from build123d import *

# Parameters (mm, degrees)
SKETCH1_W                    = 62.75
SKETCH1_H                    = 45.15
BOSS_EXTRUDE1_DEPTH          = 23.4
SKETCH2_W                    = 30
SKETCH2_H                    = 42.9
CUT_EXTRUDE1_DEPTH           = 0.95
SKETCH3_W                    = 15
SKETCH3_H                    = 13.4
CUT_EXTRUDE2_DEPTH           = 4.3
SKETCH4_R                    = 3.5
BOSS_EXTRUDE2_DEPTH          = 3
CUT_EXTRUDE3_DEPTH           = 18.6
SKETCH6_W                    = 0.2
SKETCH6_H                    = 5
CUT_EXTRUDE_THIN1_DEPTH      = 1.95
CUT_EXTRUDE_THIN1_DEPTH_BACK = 1
CUT_EXTRUDE4_DEPTH           = 5.8
SKETCH8_R                    = 2.25
CUT_EXTRUDE5_DEPTH           = 5.8
SKETCH9_W                    = 1.525
SKETCH9_H                    = 45.15
CUT_EXTRUDE6_DEPTH           = 20
SKETCH11_W                   = 1.525
SKETCH11_H                   = 10.4
BOSS_EXTRUDE3_DEPTH          = 1.4
CHAMFER1_SIZE                = 1
SKETCH10_W                   = 3
SKETCH10_H                   = 8.15
CUT_EXTRUDE7_DEPTH           = 3.75


with BuildPart() as part:
    # Sketch1 → Boss-Extrude1 (new body)
    with BuildSketch(Plane(origin=(0, 0, 0), x_dir=(1, 0, 0), z_dir=(0, 1, 0))):
        Rectangle(SKETCH1_W, SKETCH1_H)
    extrude(amount=BOSS_EXTRUDE1_DEPTH)

    # Sketch2 → Cut-Extrude1 (cut)
    with BuildSketch(Plane(origin=(0, 23.4, 0), x_dir=(1, 0, 0), z_dir=(0, 1, 0))):
        Rectangle(SKETCH2_W, SKETCH2_H)
    extrude(amount=-CUT_EXTRUDE1_DEPTH, mode=Mode.SUBTRACT)

    # Sketch3 → Cut-Extrude2 (cut)
    with BuildSketch(Plane(origin=(0, 23.4, 0), x_dir=(1, 0, 0), z_dir=(0, 1, 0))):
        with Locations((-23.875, 12.925)):
            Rectangle(SKETCH3_W, SKETCH3_H)
        with Locations((-23.875, -12.925)):
            Rectangle(SKETCH3_W, SKETCH3_H)
        with Locations((23.875, -12.925)):
            Rectangle(SKETCH3_W, SKETCH3_H)
        with Locations((23.875, 12.925)):
            Rectangle(SKETCH3_W, SKETCH3_H)
    extrude(amount=-CUT_EXTRUDE2_DEPTH, mode=Mode.SUBTRACT)

    # Sketch4 → Boss-Extrude2 (add)
    with BuildSketch(Plane(origin=(0, 19.1, 0), x_dir=(1, 0, 0), z_dir=(0, 1, 0))):
        with Locations((-23.875, 12.925)):
            Circle(SKETCH4_R)
        with Locations((-23.875, -12.925)):
            Circle(SKETCH4_R)
        with Locations((23.875, -12.925)):
            Circle(SKETCH4_R)
        with Locations((23.875, 12.925)):
            Circle(SKETCH4_R)
    extrude(amount=BOSS_EXTRUDE2_DEPTH)

    # Sketch5 → Cut-Extrude3 (cut)
    with BuildSketch(Plane(origin=(0, 23.4, 0), x_dir=(1, 0, 0), z_dir=(0, 1, 0))):
        with BuildLine():
            Line((31.375, -5.2), (23.175, -5.2))
            ThreePointArc((23.175, -5.2), (17.975, 0), (23.175, 5.2))
            Line((23.175, 5.2), (31.375, 5.2))
            ThreePointArc((31.375, 5.2), (36.575, 0), (31.375, -5.2))
        make_face()
        with BuildLine():
            Line((-31.375, 5.2), (-24.325, 5.2))
            ThreePointArc((-24.325, 5.2), (-19.125, 0), (-24.325, -5.2))
            Line((-24.325, -5.2), (-31.375, -5.2))
            ThreePointArc((-31.375, -5.2), (-36.575, 0), (-31.375, 5.2))
        make_face()
    extrude(amount=-CUT_EXTRUDE3_DEPTH, mode=Mode.SUBTRACT)

    # Sketch6 → Cut-Extrude-Thin1 (cut, two sides)
    with BuildSketch(Plane(origin=(0, 22.45, 0), x_dir=(1, 0, 0), z_dir=(0, 1, 0))) as cut_extrude_thin1_sk:
        with Locations((13.9, 0)):
            Rectangle(SKETCH6_W, SKETCH6_H)
    extrude(amount=CUT_EXTRUDE_THIN1_DEPTH, mode=Mode.SUBTRACT)
    extrude(cut_extrude_thin1_sk.sketch, amount=-CUT_EXTRUDE_THIN1_DEPTH_BACK, mode=Mode.SUBTRACT)

    # Sketch7 → Cut-Extrude4 (cut, through all)
    with BuildSketch(Plane(origin=(0, 4.8, 0), x_dir=(1, 0, 0), z_dir=(0, 1, 0))):
        with BuildLine():
            Line((22.275, 2.25), (25.075, 2.25))
            ThreePointArc((25.075, 2.25), (27.325, 0), (25.075, -2.25))
            Line((25.075, -2.25), (22.275, -2.25))
            ThreePointArc((22.275, -2.25), (20.025, 0), (22.275, 2.25))
        make_face()
    extrude(amount=-CUT_EXTRUDE4_DEPTH, mode=Mode.SUBTRACT)

    # Sketch8 → Cut-Extrude5 (cut, through all)
    with BuildSketch(Plane(origin=(0, 4.8, 0), x_dir=(1, 0, 0), z_dir=(0, 1, 0))):
        with Locations((-23.825, 0)):
            Circle(SKETCH8_R)
    extrude(amount=-CUT_EXTRUDE5_DEPTH, mode=Mode.SUBTRACT)

    # Sketch9 → Cut-Extrude6 (cut)
    with BuildSketch(Plane(origin=(0, 23.4, 0), x_dir=(1, 0, 0), z_dir=(0, 1, 0))):
        with Locations((-30.6125, 0)):
            Rectangle(SKETCH9_W, SKETCH9_H)
        with Locations((30.6125, 0)):
            Rectangle(SKETCH9_W, SKETCH9_H)
    extrude(amount=-CUT_EXTRUDE6_DEPTH, mode=Mode.SUBTRACT)

    # Sketch11 → Boss-Extrude3 (add)
    with BuildSketch(Plane(origin=(0, 3.4, 0), x_dir=(1, 0, 0), z_dir=(0, 1, 0))):
        with Locations((-30.6125, 0)):
            Rectangle(SKETCH11_W, SKETCH11_H)
        with Locations((30.6125, 0)):
            Rectangle(SKETCH11_W, SKETCH11_H)
    extrude(amount=BOSS_EXTRUDE3_DEPTH)

    # Chamfer1
    chamfer1_edges = [part.edges().sort_by_distance(p)[0] for p in [
        (-31.375, 4.8, 0),
        (31.375, 4.8, 0),
    ]]
    chamfer(chamfer1_edges, length=CHAMFER1_SIZE)

    # Sketch10 → Cut-Extrude7 (cut)
    with BuildSketch(Plane.XZ):
        with Locations((29.875, 0)):
            Rectangle(SKETCH10_W, SKETCH10_H)
        with Locations((-29.875, 0)):
            Rectangle(SKETCH10_W, SKETCH10_H)
    extrude(amount=-CUT_EXTRUDE7_DEPTH, mode=Mode.SUBTRACT)


solid = part.part
For this review, take the finished solid that the model builds, in its own axes (mm). A direction names the side the tool comes from. Coordinates: 2 decimals unless noted, no trailing zeros. Order: outer loops, then holes, each group sorted by start corner. A loop starts at its lowest first (then second) coordinate and runs counter-clockwise, first axis right, second up. Notation, with made-up numbers: (38, 1) -> (58, 1) arc R13 ccw to (58, 17) -> close; hole circle Ø4 at (75, 33.5). An arc over 180 degrees is marked (long way). Return JSON: item names as keys, results as strings.
1. We need section A-A on z = 0. State how many separate pieces and enclosed holes the cut face has, and give its area (3 significant figures).
Answer block:
{"separate pieces": "3", "enclosed holes": "0", "area": "882 mm²"}
2. We need section D-D on z = -10.5. Write out the cut boundary in (x, y) (3 decimals).
Answer block:
{"outline": "(-31.375, 0) -> (31.375, 0) -> (31.375, 3.4) -> (29.85, 3.4) -> (29.85, 19.1) -> (26.399, 19.1) -> (26.399, 22.1) -> (21.351, 22.1) -> (21.351, 19.1) -> (16.375, 19.1) -> (16.375, 23.4) -> (15, 23.4) -> (15, 22.45) -> (-15, 22.45) -> (-15, 23.4) -> (-16.375, 23.4) -> (-16.375, 19.1) -> (-21.351, 19.1) -> (-21.351, 22.1) -> (-26.399, 22.1) -> (-26.399, 19.1) -> (-29.85, 19.1) -> (-29.85, 3.4) -> (-31.375, 3.4) -> close"}
3. We need section B-B on y = 7.25. Write out the cut boundary in (x, z) (3 decimals), and give its area (3 significant figures).
Answer block:
{"outline": "(-29.85, -22.575) -> (29.85, -22.575) -> (29.85, -5.2) -> (23.175, -5.2) arc R5.2 cw to (23.175, 5.2) -> (29.85, 5.2) -> (29.85, 22.575) -> (-29.85, 22.575) -> (-29.85, 5.2) -> (-24.325, 5.2) arc R5.2 cw to (-24.325, -5.2) -> (-29.85, -5.2) -> close", "area": "2,480 mm²"}
4. The part is to be moulded in two halves that separate along Z. For faces 1 (the flat face through (0, 12, -22.575)), 2 (the cylindrical face through (17.976, 14.23, 0.114)), 3 (the flat face through (31, 3.4, 14)), say which applies: +Z half, -Z half, draft (parallel to the pull), parting line (faces both ways), or undercut.
Answer block:
{"face 1": "-Z half", "face 2": "undercut", "face 3": "draft"}
5. We need section C-C on x = 9.5. Write out the cut boundary in (y, z) (3 decimals).
Answer block:
{"outline": "(0, -22.575) -> (23.4, -22.575) -> (23.4, -21.45) -> (22.45, -21.45) -> (22.45, 21.45) -> (23.4, 21.45) -> (23.4, 22.575) -> (0, 22.575) -> close"}
6. For line 1 (X direction, y = 2.35, z = 0) (3 decimals); line 2 (Z direction, x = -25, y = 6) (3 decimals); line 3 (Z direction, x = 22, y = 21) (1 decimal), list the stretches that pass through material, from the lowest coordinate up. Write a range as from..to.
Answer block:
{"line 1": "-28.375..-26.075, -21.575..20.025, 27.325..28.375", "line 2": "-22.575..-5.2, 5.2..22.575", "line 3": "-22.6..-19.6, -15.9..-10, -6.2..-5.1, 5.1..6.2, 10..15.9, 19.6..22.6"}
7. For pin 1 Ø5.5 at (x, z) = (25, -12) entering from +Y; pin 2 Ø5 at (y, z) = (18, 10) entering from -X; pin 3 Ø1.7 at (x, z) = (-30, 10.5) entering from +Y, all flat-tipped, find the tip position at first contact; note any pin that passes through.
Answer block:
{"pin 1": "y = 22.1", "pin 2": "x = -29.85", "pin 3": "y = 19.1"}
8. Machinability: for faces 4 (the flat face through (-30, 2, 4.075)), 5 (the flat face through (-31, 3.4, 14)), 6 (the flat face through (24, 2, 2.25)), 7 (the flat face through (23, 21, 19.625)), 8 (the flat face through (-16.375, 21, -13)), which of the approach directions +Z, -Z, +X, -X, +Y, -Y give a long, thin tool a straight path to every point of the face, cutting with its end or side? Answer none if there is none.
Answer block:
{"face 4": "-X, -Y", "face 5": "+Z, -X, +Y", "face 6": "+Y, -Y", "face 7": "+X, +Y", "face 8": "+Y"}
